Verification items for the finished model (mm, model axes). A direction names the side the tool comes from. Give positions to 0.01 mm unless a question says otherwise; leave off trailing zeros. Order: outer loops, then holes, each group sorted by start corner. A loop starts at its lowest first (then second) coordinate and runs counter-clockwise, first axis right, second up. Notation, with made-up numbers: (73.5, -38.5) - (109.5, -38.5) arc R12 cw to (109.5, -30.5) - close; hole circle Ø7 at (25.5, 76.5). An arc over 180 degrees is marked (long way). Answer as a JSON object with one key per item and string values.
```python
from build123d import *

# Parameters (mm, degrees)
SKETCH1_W           = 7
SKETCH1_H           = 56.5
BOSS_EXTRUDE1_DEPTH = 3
SKETCH2_W           = 2.8
SKETCH2_H           = 19
BOSS_EXTRUDE2_DEPTH = 1
SKETCH3_W           = 7
SKETCH3_H           = 2.85
SKETCH3_H_2         = 1.35
BOSS_EXTRUDE3_DEPTH = 4
SKETCH4_W           = 3
SKETCH4_H           = 18
BOSS_EXTRUDE4_DEPTH = 5
SKETCH5_W           = 3
SKETCH5_H           = 18
BOSS_EXTRUDE5_DEPTH = 5
SKETCH9_R           = 5.85
BOSS_EXTRUDE7_DEPTH = 8
FILLET1_R           = 1.5
FILLET2_R           = 1
SKETCH11_R          = 3.436863838
SKETCH7_R           = 1.6
CUT_EXTRUDE5_START  = -2
CUT_EXTRUDE5_DEPTH  = 2
SKETCH14_R          = 1.6
CUT_EXTRUDE6_DEPTH  = 3


with BuildPart() as part:
    # Sketch1 → Boss-Extrude1 (new body)
    with BuildSketch(Plane.XY):
        with Locations((0, 9.795104227)):
            Rectangle(SKETCH1_W, SKETCH1_H)
    extrude(amount=BOSS_EXTRUDE1_DEPTH)

    # Sketch2 → Boss-Extrude2 (add)
    with BuildSketch(Plane.XY.offset(3)):
        with Locations((0, 18.995104227)):
            Rectangle(SKETCH2_W, SKETCH2_H)
    extrude(amount=BOSS_EXTRUDE2_DEPTH)

    # Sketch3 → Boss-Extrude3 (add)
    with BuildSketch(Plane.XY.offset(3)):
        with Locations((0, 36.620104227)):
            Rectangle(SKETCH3_W, SKETCH3_H)
        with Locations((0, -17.779895773)):
            Rectangle(SKETCH3_W, SKETCH3_H_2)
    extrude(amount=BOSS_EXTRUDE3_DEPTH)

    # Sketch4 → Boss-Extrude4 (add)
    with BuildSketch(Plane.ZY.offset(3.5)):
        with Locations((1.5, 29.045104227)):
            Rectangle(SKETCH4_W, SKETCH4_H)
    extrude(amount=BOSS_EXTRUDE4_DEPTH)

    # Sketch5 → Boss-Extrude5 (add)
    with BuildSketch(Plane(origin=(3.5, 0, 0), x_dir=(0, 0, -1), z_dir=(1, 0, 0))):
        with Locations((-1.5, 29.045104227)):
            Rectangle(SKETCH5_W, SKETCH5_H)
    extrude(amount=BOSS_EXTRUDE5_DEPTH)

    # Sketch9 → Boss-Extrude7 (add)
    with BuildSketch(Plane(origin=(0, 0, 0), x_dir=(-1, 0, 0), z_dir=(0, 0, -1))):
        with Locations(Location((0, 26.670104227, 0), (0, 0, 180))):
            Circle(SKETCH9_R)
    extrude(amount=BOSS_EXTRUDE7_DEPTH)

    # Fillet1
    fillet1_edges = [part.edges().sort_by_distance(p)[0] for p in [
        (-5.85, 26.670104227, -8),
    ]]
    fillet(fillet1_edges, radius=FILLET1_R)

    # Fillet2
    fillet2_edges = [part.edges().sort_by_distance(p)[0] for p in [
        (-3.5, 20.045104227, 1.5),
        (-8.5, 20.045104227, 1.5),
        (-8.5, 38.045104227, 1.5),
        (3.5, 20.045104227, 1.5),
        (8.5, 38.045104227, 1.5),
        (8.5, 20.045104227, 1.5),
    ]]
    fillet(fillet2_edges, radius=FILLET2_R)

    # Sketch11 → Cut-Loft6 section 0
    with BuildSketch(Plane(origin=(0, 0, -8), x_dir=(-1, 0, 0), z_dir=(0, 0, -1))):
        with Locations((0, 26.670104227)):
            Circle(SKETCH11_R)
    # Sketch7 → Cut-Loft6 section 1
    with BuildSketch(Plane.XY.offset(3)):
        with Locations((0, 29.495104227)):
            Circle(SKETCH7_R)
    loft(mode=Mode.SUBTRACT)

    # Cut-Extrude5: read off the stored shape, not the designer's step
    # Cut-Extrude5 outline → Cut-Extrude5 (cut)
    with BuildSketch(Plane(origin=(0, 0, -8), x_dir=(-1, 0, 0), z_dir=(0, 0, -1)).offset(CUT_EXTRUDE5_START)):
        with BuildLine():
            ThreePointArc((5.066248612, 29.595104227), (2.925, 31.736352839), (0, 32.520104227))
            Line((0, 32.520104227), (0, 26.670104227))
            Line((0, 26.670104227), (5.066248612, 29.595104227))
        make_face()
        with BuildLine():
            Line((0, 26.670104227), (-5.066248612, 29.595104227))
            ThreePointArc((-5.066248612, 29.595104227), (-5.85, 26.670104227), (-5.066248612, 23.745104227))
            Line((-5.066248612, 23.745104227), (0, 26.670104227))
        make_face()
        with BuildLine():
            Line((5.066248612, 23.745104227), (0, 26.670104227))
            Line((0, 26.670104227), (0, 20.820104227))
            ThreePointArc((0, 20.820104227), (2.925, 21.603855615), (5.066248612, 23.745104227))
        make_face()
    extrude(amount=CUT_EXTRUDE5_DEPTH, mode=Mode.SUBTRACT)

    # Sketch14 → Cut-Extrude6 (cut)
    with BuildSketch(Plane.XY.offset(3)):
        with Locations((0, 29.495104227)):
            Circle(SKETCH14_R)
    extrude(amount=CUT_EXTRUDE6_DEPTH, mode=Mode.SUBTRACT)


solid = part.part
```
(1) Release check for a two-part mould opening along Y. For faces 5 (the flat face through (-2, 23, -6)), 6 (the flat face through (1.4, 18.9, 3.5)), 7 (the cylindrical face through (-8.2, 37.76, 1.52)), 8 (the flat face through (0, -18.455, 3)) record: pulls with the +Y half, pulls with the -Y half, needs draft (parallel to the pull), parting line crosses it, or undercut.
Computed values:
{"face 5": "needs draft", "face 6": "undercut", "face 7": "pulls with the +Y half", "face 8": "pulls with the -Y half"}
(2) Section check C-C (y = 4.5). Record the cut outline in (x, z).
Computed values:
{"outline": "(-3.5, 0) - (3.5, 0) - (3.5, 3) - (-3.5, 3) - close"}
(3) Gauge pin test, flat ends, axial feed: pin 1 Ø3.5 at (x, y) = (-2, 31.5) entering from -Z; pin 2 Ø5 at (x, y) = (2, 10.5) entering from -Z; pin 3 Ø0.9 at (y, z) = (37, 5) entering from -X; pin 4 Ø2 at (y, z) = (-8.5, 4.5) entering from +X. Record the tip position at first contact, or that the pin passes through.
Computed values:
{"pin 1": "stops at z = -6", "pin 2": "stops at z = 0", "pin 3": "stops at x = -3.5", "pin 4": "passes through"}
(4) Material ranges on line 1 along Y through (x, z) = (1, 5); line 2 along Y through (x, z) = (-6.5, 2.75); line 3 along X through (y, z) = (11.5, 3.5), recorded low to high. Write a range as [from, to].
Computed values:
{"line 1": "y = [-18.45, -17.1], [35.2, 38.05]", "line 2": "y = [20.05, 38.05]", "line 3": "x = [-1.4, 1.4]"}
(5) Access from +Z, -Z, +X, -X, +Y, -Y to the whole of each face (thin tool, end or side, straight path). Record for faces 1 (the flat face through (3.5, 37, 5)), 2 (the flat face through (3.959, 28.956, -6.986)), 3 (the flat face through (-1.4, 18.9, 3.5)), 4 (the flat face through (0, 9.495, 3.5)).
Computed values:
{"face 1": "+Z, +X, +Y, -Y", "face 2": "-Z, +X", "face 3": "+Z, -X", "face 4": "+Z, +X, -X"}
(6) Section check B-B (x = -7). Record the cut outline in (y, z), then the cut area to 3 significant figures.
Computed values:
{"outline": "(20.05, 0) - (38.05, 0) - (38.05, 3) - (20.05, 3) - close", "area": "54.0 mm²"}
(7) Section check A-A (y = 12). Record the cut outline in (x, z).
Computed values:
{"outline": "(-3.5, 0) - (3.5, 0) - (3.5, 3) - (1.4, 3) - (1.4, 4) - (-1.4, 4) - (-1.4, 3) - (-3.5, 3) - close"}
